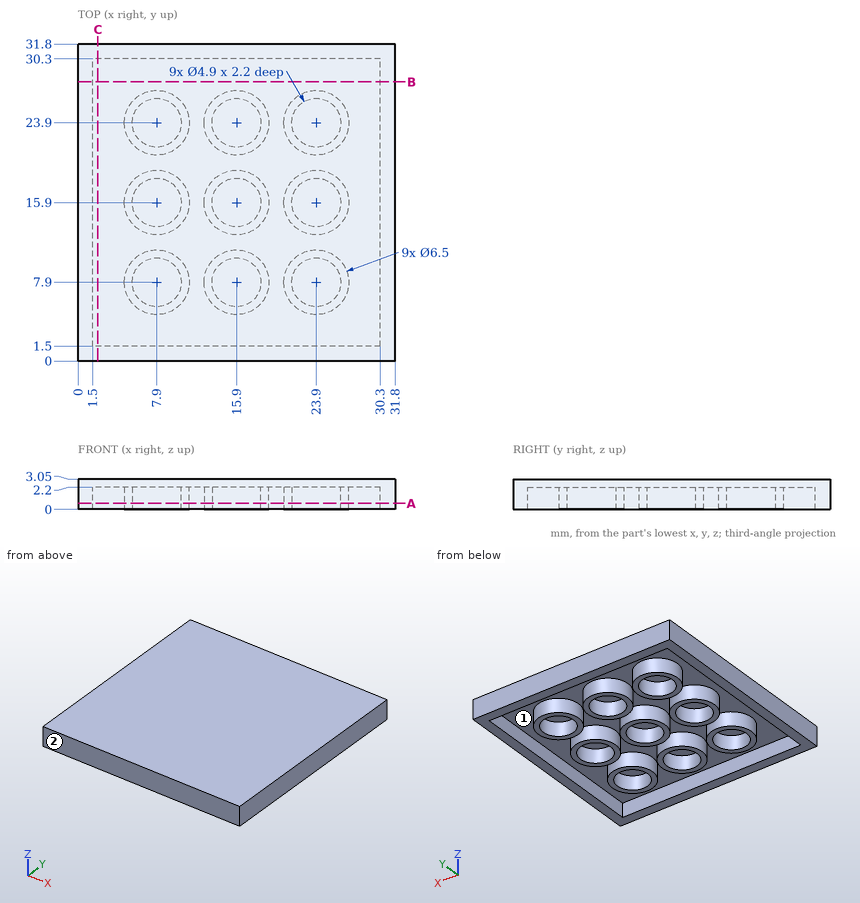
Drawing for the job (mm, zero at the part's lowest x, y, z). Round coordinates to 2 decimals unless told otherwise and drop trailing zeros. Write each loop counter-clockwise with the first axis right and the second up, starting at its lowest first coordinate (ties: lowest second). Pieces come first, ordered by that corner, then holes. Notation, with made-up numbers: (63.5, -33) - (73.5, -33) arc R28 cw to (73.5, -15) - close; hole circle Ø9 at (-28, 23). An arc over 180 degrees is marked (long way). Return JSON: item names as keys, results as strings. Group by question number.
Item 1: Probe probe 1 along Y at (x, z) = (29, 1.6); probe 2 along X at (y, z) = (13, 0.75); probe 3 along Z at (x, y) = (24, 12.5). List the from-to ranges inside material, lowest first.
Item 2: Mould opens along X. For the marked faces 1 and 2 say: +X half, -X half, draft (parallel to the pull), parting line (faces both ways), or undercut.
Item 3: Band-saw the part on B-B on y = 28. List the corners of the cut face in (x, z).
Item 4: Flat gauge pin, fed straight in: pin 1 Ø3 at (x, y) = (7.9, 7.9) entering from -Z. Where does the tip first touch, or does it go through?
Item 5: Band-saw the part on A-A on z = 0.6. State how many separate pieces and enclosed holes the cut face has, plus the area to 3 significant figures.
Resolved:
{
 "1": {"probe 1": "y = 0 to 1.5, 30.3 to 31.8", "probe 2": "x = 0 to 1.5, 6.43 to 9.37, 14.43 to 17.37, 22.43 to 25.37, 30.3 to 31.8", "probe 3": "z = 2.2 to 3.05"},
 "2": {"face 1": "undercut", "face 2": "draft"},
 "3": {"outline": "(0, 0) - (1.5, 0) - (1.5, 2.2) - (30.3, 2.2) - (30.3, 0) - (31.8, 0) - (31.8, 3.05) - (0, 3.05) - close"},
 "4": {"pin 1": "stops at z = 2.2"},
 "5": {"separate pieces": "10", "enclosed holes": "10", "area": "311 mm²"}
}
